Here's how the part is built. I have some questions about the finished solid (model axes, mm). Face numbers are marked on the shaded views. A direction names the side the tool comes from. Give positions to 0.01 mm unless a question says otherwise; leave off trailing zeros. Loops run counter-clockwise (first coordinate to the right, second up) from the corner with the lowest first, then second, coordinate; pieces in that order, holes last.
Q1. Thinking about a two-plate mould opening in Z: for the marked faces 4, 5 and 6, which applies, pulls with the +Z half, pulls with the -Z half, needs draft (parallel to the pull), parting line crosses it, or undercut?
Q2. Suppose I cut it at C-C (y = -8.5). List the corners of the cut face in (x, z) for me.
Q3. I need wall thicknesses on probe 1 along X at (y, z) = (0.25, -58); probe 2 along X at (y, z) = (4.85, -5); probe 3 along Y at (x, z) = (-5.5, -63). Which ranges of each line are inside material? Lowest first, please.
Q4. Suppose I cut it at D-D (x = -10). List the corners of the cut face in (y, z) for me, and give its area (3 significant figures).
Q5. Suppose I cut it at B-B (x = 0). List the corners of the cut face in (y, z) for me, and give its area (3 significant figures).
Q6. Suppose I cut it at A-A (y = 0). List the corners of the cut face in (x, z) for me, and give its area (3 significant figures).
Q7. For the marked faces 1, 2 and 3, which set-ups out of +Z, -Z, +X, -X, +Y, -Y let a thin tool reach every point of the face, with its end or its side?
Q8. I'm going to push flat-ended pins straight in: P1, Ø20, axis at x = 2, z = -57.5, coming from the -Y side; P2, Ø4, axis at y = -7, z = -68.5, coming from the +X side; P3, Ø9, axis at x = -5, z = 5, coming from the -Y side; P4, Ø2.5, axis at x = -10, y = -8.5, coming from the -Z side. Where does each tip first touch, or does it pass through?
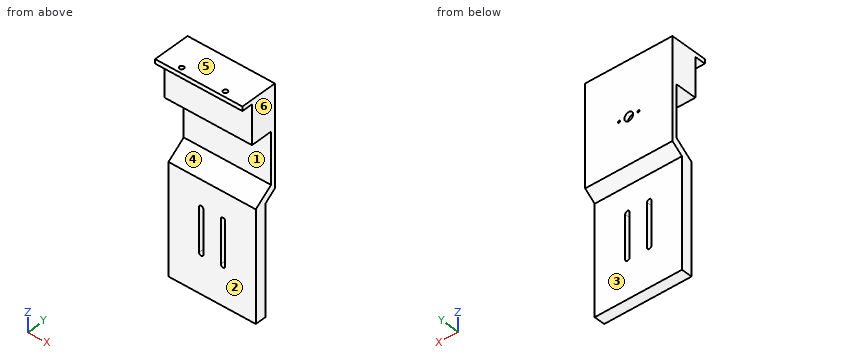
```python
from build123d import *

# Parameters (mm, degrees)
SKETCH_1_W          = 40
SKETCH_1_H          = 12
EXTRUDE_1_DEPTH     = 20
SKETCH_2_W          = 40
SKETCH_2_H          = 2
EXTRUDE_2_DEPTH     = 23.5
SKETCH_3_W          = 40
SKETCH_3_H          = 2
EXTRUDE_3_DEPTH     = 5
CUT_EXTRUDE_1_REACH = 19
SKETCH_4_R          = 0.5
SKETCH_4_R_2        = 2
CUT_EXTRUDE_2_REACH = 4
SKETCH_5_R          = 1
EXTRUDE_4_DEPTH     = 40
CUT_EXTRUDE_3_DEPTH = 40
CUT_EXTRUDE_5_REACH = 14


with BuildPart() as part:
    # 草图1 → 凸台-拉伸1 (new body)
    with BuildSketch(Plane.XY):
        Rectangle(SKETCH_1_W, SKETCH_1_H)
    extrude(amount=EXTRUDE_1_DEPTH)

    # 草图2 → 凸台-拉伸2 (add)
    with BuildSketch(Plane(origin=(0, 0, 0), x_dir=(-1, 0, 0), z_dir=(0, 0, -1))):
        with Locations((0, 5)):
            Rectangle(SKETCH_2_W, SKETCH_2_H)
    extrude(amount=EXTRUDE_2_DEPTH)

    # 草图3 → 凸台-拉伸3 (add)
    with BuildSketch(Plane.XZ.offset(6)):
        with Locations((0, 19)):
            Rectangle(SKETCH_3_W, SKETCH_3_H)
    extrude(amount=EXTRUDE_3_DEPTH)

    # 草图4 → 切除-拉伸1 (cut, up to next)
    with BuildSketch(Plane(origin=(0, 6, 0), x_dir=(1, 0, 0), z_dir=(0, 1, 0)), mode=Mode.PRIVATE) as cut_extrude_1_sk1:
        with Locations((-4.5, 5)):
            Circle(SKETCH_4_R)
    cut_extrude_1_tool1 = extrude(cut_extrude_1_sk1.sketch, amount=-CUT_EXTRUDE_1_REACH, mode=Mode.PRIVATE) & part.part
    add(cut_extrude_1_tool1.solids().sort_by_distance((-4.5, 6, -5))[0], mode=Mode.SUBTRACT)
    # 草图4 → 切除-拉伸1 (cut, up to next)
    with BuildSketch(Plane(origin=(0, 6, 0), x_dir=(1, 0, 0), z_dir=(0, 1, 0)), mode=Mode.PRIVATE) as cut_extrude_1_sk2:
        with Locations((4.5, 5)):
            Circle(SKETCH_4_R)
    cut_extrude_1_tool2 = extrude(cut_extrude_1_sk2.sketch, amount=-CUT_EXTRUDE_1_REACH, mode=Mode.PRIVATE) & part.part
    add(cut_extrude_1_tool2.solids().sort_by_distance((4.5, 6, -5))[0], mode=Mode.SUBTRACT)
    # 草图4 → 切除-拉伸1 (cut, up to next)
    with BuildSketch(Plane(origin=(0, 6, 0), x_dir=(1, 0, 0), z_dir=(0, 1, 0)), mode=Mode.PRIVATE) as cut_extrude_1_sk3:
        with Locations((0, 5)):
            Circle(SKETCH_4_R_2)
    cut_extrude_1_tool3 = extrude(cut_extrude_1_sk3.sketch, amount=-CUT_EXTRUDE_1_REACH, mode=Mode.PRIVATE) & part.part
    add(cut_extrude_1_tool3.solids().sort_by_distance((0, 6, -5))[0], mode=Mode.SUBTRACT)

    # 草图5 → 切除-拉伸2 (cut, up to next)
    with BuildSketch(Plane(origin=(0, 0, 18), x_dir=(-1, 0, 0), z_dir=(0, 0, -1)), mode=Mode.PRIVATE) as cut_extrude_2_sk1:
        with Locations((-10, -8.5)):
            Circle(SKETCH_5_R)
    cut_extrude_2_tool1 = extrude(cut_extrude_2_sk1.sketch, amount=-CUT_EXTRUDE_2_REACH, mode=Mode.PRIVATE) & part.part
    add(cut_extrude_2_tool1.solids().sort_by_distance((10, -8.5, 18))[0], mode=Mode.SUBTRACT)
    # 草图5 → 切除-拉伸2 (cut, up to next)
    with BuildSketch(Plane(origin=(0, 0, 18), x_dir=(-1, 0, 0), z_dir=(0, 0, -1)), mode=Mode.PRIVATE) as cut_extrude_2_sk2:
        with Locations((10, -8.5)):
            Circle(SKETCH_5_R)
    cut_extrude_2_tool2 = extrude(cut_extrude_2_sk2.sketch, amount=-CUT_EXTRUDE_2_REACH, mode=Mode.PRIVATE) & part.part
    add(cut_extrude_2_tool2.solids().sort_by_distance((-10, -8.5, 18))[0], mode=Mode.SUBTRACT)

    # 草图6 → 凸台-拉伸4 (add)
    with BuildSketch(Plane(origin=(20, 0, 0), x_dir=(0, 0, -1), z_dir=(1, 0, 0))):
        Polygon((23.5, 4), (29.5, -4), (80, -4), (80, 6), (23.5, 6), align=None)
    extrude(amount=-EXTRUDE_4_DEPTH)

    # 草图7 → 切除-拉伸3 (cut)
    with BuildSketch(Plane.ZY.offset(20)):
        Polygon((-30, 1), (-26.25, 6), (-80, 6), (-80, 1), align=None)
    extrude(amount=-CUT_EXTRUDE_3_DEPTH, mode=Mode.SUBTRACT)

    # 草图9 → 切除-拉伸5 (cut, up to next)
    with BuildSketch(Plane(origin=(0, 1, 0), x_dir=(1, 0, 0), z_dir=(0, 1, 0)), mode=Mode.PRIVATE) as cut_extrude_5_sk1:
        with BuildLine():
            Line((-4, 62), (-4, 42))
            ThreePointArc((-4, 42), (-5, 41), (-6, 42))
            Line((-6, 42), (-6, 62))
            ThreePointArc((-6, 62), (-5, 63), (-4, 62))
        make_face()
    cut_extrude_5_tool1 = extrude(cut_extrude_5_sk1.sketch, amount=-CUT_EXTRUDE_5_REACH, mode=Mode.PRIVATE) & part.part
    add(cut_extrude_5_tool1.solids().sort_by_distance((-5, 1, -52))[0], mode=Mode.SUBTRACT)
    # 草图9 → 切除-拉伸5 (cut, up to next)
    with BuildSketch(Plane(origin=(0, 1, 0), x_dir=(1, 0, 0), z_dir=(0, 1, 0)), mode=Mode.PRIVATE) as cut_extrude_5_sk2:
        with BuildLine():
            Line((4, 62), (4, 42))
            ThreePointArc((4, 42), (5, 41), (6, 42))
            Line((6, 42), (6, 62))
            ThreePointArc((6, 62), (5, 63), (4, 62))
        make_face()
    cut_extrude_5_tool2 = extrude(cut_extrude_5_sk2.sketch, amount=-CUT_EXTRUDE_5_REACH, mode=Mode.PRIVATE) & part.part
    add(cut_extrude_5_tool2.solids().sort_by_distance((5, 1, -52))[0], mode=Mode.SUBTRACT)


solid = part.part
```
Solutions:
1. face 4: undercut
1. face 5: pulls with the +Z half
1. face 6: needs draft
2. outline: (-20, 18) - (-11, 18) - (-11, 20) - (-20, 20) - close; (-9, 18) - (9, 18) - (9, 20) - (-9, 20) - close; (11, 18) - (20, 18) - (20, 20) - (11, 20) - close
3. probe 1: x = -20 to -6, -4 to 4, 6 to 20
3. probe 2: x = -20 to -5, -4 to -2, 2 to 4, 5 to 20
3. probe 3: y = -4 to 1
4. outline: (-11, 18) - (-9.5, 18) - (-9.5, 20) - (-11, 20) - close; (-7.5, 18) - (-6, 18) - (-6, 0) - (4, 0) - (4, -23.5) - (-4, -29.5) - (-4, -80) - (1, -80) - (1, -30) - (6, -26.25) - (6, 20) - (-7.5, 20) - close
4. area: 575 mm2
5. outline: (-11, 18) - (-6, 18) - (-6, 0) - (4, 0) - (4, -3) - (6, -3) - (6, 20) - (-11, 20) - close; (-4, -80) - (1, -80) - (1, -30) - (6, -26.25) - (6, -7) - (4, -7) - (4, -23.5) - (-4, -29.5) - close
5. area: 571 mm2
6. outline: (-20, -80) - (20, -80) - (20, -26.5) - (-20, -26.5) - close; (-20, 0) - (20, 0) - (20, 20) - (-20, 20) - close; hole (-6, -62) arc R1 ccw to (-4, -62) - (-4, -42) arc R1 ccw to (-6, -42) - close; hole (4, -62) arc R1 ccw to (6, -62) - (6, -42) arc R1 ccw to (4, -42) - close
6. area: 2,850 mm2
7. face 1: +X, -X, -Y
7. face 2: -Z, +X, -X, -Y
7. face 3: -Z, +X, -X, +Y
8. P1: stops at y = -4
8. P2: passes through
8. P3: stops at y = -6
8. P4: stops at z = 18
